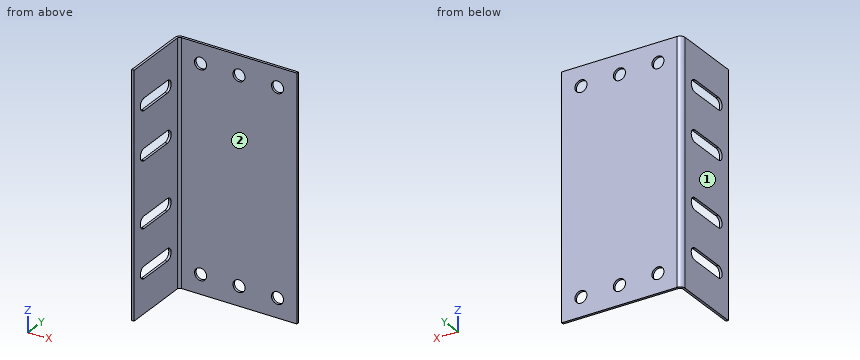
from build123d import *

# Parameters (mm, degrees)
BASE_FLANGE1_DEPTH = 100
CUT_EXTRUDE3_REACH = 117.758
SKETCH8_R          = 2.5
CUT_EXTRUDE4_REACH = 117.758
SKETCH11_R         = 2.5


# Sheet-metal steps are written as plain solids
with BuildPart() as part:
    # Sketch2 → Base-Flange1 (new body)
    with BuildSketch(Plane.XY):
        with BuildLine():
            Line((0, 0), (0, 28))
            ThreePointArc((0, 28), (0.585786438, 29.414213562), (2, 30))
            Line((2, 30), (50, 30))
            Line((50, 30), (50, 29))
            Line((50, 29), (2, 29))
            ThreePointArc((2, 29), (1.292893219, 28.707106781), (1, 28))
            Line((1, 28), (1, 0))
            Line((1, 0), (0, 0))
        make_face()
    extrude(amount=BASE_FLANGE1_DEPTH)

    # Sketch8 → Cut-Extrude3 (cut, up to next)
    with BuildSketch(Plane(origin=(0, 30, 0), x_dir=(1, 0, 0), z_dir=(0, 1, 0)), mode=Mode.PRIVATE) as cut_extrude3_sk1:
        with Locations(Location((42, -8, 0), (0, 0, 270))):
            Circle(SKETCH8_R)
    cut_extrude3_tool1 = extrude(cut_extrude3_sk1.sketch, amount=-CUT_EXTRUDE3_REACH, mode=Mode.PRIVATE) & part.part
    # Sketch8 → Cut-Extrude3 (cut, up to next)
    with BuildSketch(Plane(origin=(0, 30, 0), x_dir=(1, 0, 0), z_dir=(0, 1, 0)), mode=Mode.PRIVATE) as cut_extrude3_sk2:
        with Locations(Location((10, -8, 0), (0, 0, 270))):
            Circle(SKETCH8_R)
    cut_extrude3_tool2 = extrude(cut_extrude3_sk2.sketch, amount=-CUT_EXTRUDE3_REACH, mode=Mode.PRIVATE) & part.part
    # Sketch8 → Cut-Extrude3 (cut, up to next)
    with BuildSketch(Plane(origin=(0, 30, 0), x_dir=(1, 0, 0), z_dir=(0, 1, 0)), mode=Mode.PRIVATE) as cut_extrude3_sk3:
        with Locations(Location((42, -92, 0), (0, 0, 270))):
            Circle(SKETCH8_R)
    cut_extrude3_tool3 = extrude(cut_extrude3_sk3.sketch, amount=-CUT_EXTRUDE3_REACH, mode=Mode.PRIVATE) & part.part
    # Sketch8 → Cut-Extrude3 (cut, up to next)
    with BuildSketch(Plane(origin=(0, 30, 0), x_dir=(1, 0, 0), z_dir=(0, 1, 0)), mode=Mode.PRIVATE) as cut_extrude3_sk4:
        with Locations(Location((10, -92, 0), (0, 0, 270))):
            Circle(SKETCH8_R)
    cut_extrude3_tool4 = extrude(cut_extrude3_sk4.sketch, amount=-CUT_EXTRUDE3_REACH, mode=Mode.PRIVATE) & part.part
    # Sketch8 → Cut-Extrude3 (cut, up to next)
    with BuildSketch(Plane(origin=(0, 30, 0), x_dir=(1, 0, 0), z_dir=(0, 1, 0)), mode=Mode.PRIVATE) as cut_extrude3_sk5:
        with Locations(Location((26, -8, 0), (0, 0, 270))):
            Circle(SKETCH8_R)
    cut_extrude3_tool5 = extrude(cut_extrude3_sk5.sketch, amount=-CUT_EXTRUDE3_REACH, mode=Mode.PRIVATE) & part.part
    # Sketch8 → Cut-Extrude3 (cut, up to next)
    with BuildSketch(Plane(origin=(0, 30, 0), x_dir=(1, 0, 0), z_dir=(0, 1, 0)), mode=Mode.PRIVATE) as cut_extrude3_sk6:
        with Locations(Location((26, -92, 0), (0, 0, 270))):
            Circle(SKETCH8_R)
    cut_extrude3_tool6 = extrude(cut_extrude3_sk6.sketch, amount=-CUT_EXTRUDE3_REACH, mode=Mode.PRIVATE) & part.part
    add(cut_extrude3_tool1.solids().sort_by_distance((42, 30, 8))[0], mode=Mode.SUBTRACT)
    add(cut_extrude3_tool2.solids().sort_by_distance((10, 30, 8))[0], mode=Mode.SUBTRACT)
    add(cut_extrude3_tool3.solids().sort_by_distance((42, 30, 92))[0], mode=Mode.SUBTRACT)
    add(cut_extrude3_tool4.solids().sort_by_distance((10, 30, 92))[0], mode=Mode.SUBTRACT)
    add(cut_extrude3_tool5.solids().sort_by_distance((26, 30, 8))[0], mode=Mode.SUBTRACT)
    add(cut_extrude3_tool6.solids().sort_by_distance((26, 30, 92))[0], mode=Mode.SUBTRACT)

    # Sketch11 → Cut-Extrude4 (cut, up to next)
    with BuildSketch(Plane.ZY, mode=Mode.PRIVATE) as cut_extrude4_sk1:
        with BuildLine():
            ThreePointArc((19, 21.5), (16.5, 24), (14, 21.5))
            Line((14, 21.5), (14, 13.999999995))
            ThreePointArc((14, 13.999999995), (16.499999997, 16.5), (19, 14))
            Line((19, 14), (19, 21.5))
        make_face()
    cut_extrude4_tool1 = extrude(cut_extrude4_sk1.sketch, amount=-CUT_EXTRUDE4_REACH, mode=Mode.PRIVATE) & part.part
    # Sketch11 → Cut-Extrude4 (cut, up to next)
    with BuildSketch(Plane.ZY, mode=Mode.PRIVATE) as cut_extrude4_sk2:
        with BuildLine():
            ThreePointArc((19, 14), (16.500000003, 11.5), (14, 13.999999995))
            Line((14, 13.999999995), (14, 6.5))
            ThreePointArc((14, 6.5), (16.5, 4), (19, 6.5))
            Line((19, 6.5), (19, 14))
        make_face()
    cut_extrude4_tool2 = extrude(cut_extrude4_sk2.sketch, amount=-CUT_EXTRUDE4_REACH, mode=Mode.PRIVATE) & part.part
    # Sketch11 → Cut-Extrude4 (cut, up to next)
    with BuildSketch(Plane.ZY, mode=Mode.PRIVATE) as cut_extrude4_sk3:
        with Locations((16.5, 14)):
            Circle(SKETCH11_R)
    cut_extrude4_tool3 = extrude(cut_extrude4_sk3.sketch, amount=-CUT_EXTRUDE4_REACH, mode=Mode.PRIVATE) & part.part
    # Sketch11 → Cut-Extrude4 (cut, up to next)
    with BuildSketch(Plane.ZY, mode=Mode.PRIVATE) as cut_extrude4_sk4:
        with BuildLine():
            ThreePointArc((39, 14), (36.5, 11.5), (34, 14))
            Line((34, 14), (34, 6.5))
            ThreePointArc((34, 6.5), (36.5, 4), (39, 6.5))
            Line((39, 6.5), (39, 14))
        make_face()
    cut_extrude4_tool4 = extrude(cut_extrude4_sk4.sketch, amount=-CUT_EXTRUDE4_REACH, mode=Mode.PRIVATE) & part.part
    # Sketch11 → Cut-Extrude4 (cut, up to next)
    with BuildSketch(Plane.ZY, mode=Mode.PRIVATE) as cut_extrude4_sk5:
        with Locations((36.5, 14)):
            Circle(SKETCH11_R)
    cut_extrude4_tool5 = extrude(cut_extrude4_sk5.sketch, amount=-CUT_EXTRUDE4_REACH, mode=Mode.PRIVATE) & part.part
    # Sketch11 → Cut-Extrude4 (cut, up to next)
    with BuildSketch(Plane.ZY, mode=Mode.PRIVATE) as cut_extrude4_sk6:
        with BuildLine():
            ThreePointArc((39, 21.5), (36.5, 24), (34, 21.5))
            Line((34, 21.5), (34, 14))
            ThreePointArc((34, 14), (36.5, 16.5), (39, 14))
            Line((39, 14), (39, 21.5))
        make_face()
    cut_extrude4_tool6 = extrude(cut_extrude4_sk6.sketch, amount=-CUT_EXTRUDE4_REACH, mode=Mode.PRIVATE) & part.part
    # Sketch11 → Cut-Extrude4 (cut, up to next)
    with BuildSketch(Plane.ZY, mode=Mode.PRIVATE) as cut_extrude4_sk7:
        with BuildLine():
            Line((86, 14), (86, 21.5))
            ThreePointArc((86, 21.5), (83.5, 24), (81, 21.5))
            Line((81, 21.5), (81, 14))
            ThreePointArc((81, 14), (83.5, 16.5), (86, 14))
        make_face()
    cut_extrude4_tool7 = extrude(cut_extrude4_sk7.sketch, amount=-CUT_EXTRUDE4_REACH, mode=Mode.PRIVATE) & part.part
    # Sketch11 → Cut-Extrude4 (cut, up to next)
    with BuildSketch(Plane.ZY, mode=Mode.PRIVATE) as cut_extrude4_sk8:
        with BuildLine():
            Line((86, 6.5), (86, 14))
            ThreePointArc((86, 14), (83.5, 11.5), (81, 14))
            Line((81, 14), (81, 6.5))
            ThreePointArc((81, 6.5), (83.5, 4), (86, 6.5))
        make_face()
    cut_extrude4_tool8 = extrude(cut_extrude4_sk8.sketch, amount=-CUT_EXTRUDE4_REACH, mode=Mode.PRIVATE) & part.part
    # Sketch11 → Cut-Extrude4 (cut, up to next)
    with BuildSketch(Plane.ZY, mode=Mode.PRIVATE) as cut_extrude4_sk9:
        with Locations((83.5, 14)):
            Circle(SKETCH11_R)
    cut_extrude4_tool9 = extrude(cut_extrude4_sk9.sketch, amount=-CUT_EXTRUDE4_REACH, mode=Mode.PRIVATE) & part.part
    # Sketch11 → Cut-Extrude4 (cut, up to next)
    with BuildSketch(Plane.ZY, mode=Mode.PRIVATE) as cut_extrude4_sk10:
        with BuildLine():
            ThreePointArc((66, 21.5), (63.5, 24), (61, 21.5))
            Line((61, 21.5), (61, 14))
            ThreePointArc((61, 14), (63.5, 16.5), (66, 14))
            Line((66, 14), (66, 21.5))
        make_face()
    cut_extrude4_tool10 = extrude(cut_extrude4_sk10.sketch, amount=-CUT_EXTRUDE4_REACH, mode=Mode.PRIVATE) & part.part
    # Sketch11 → Cut-Extrude4 (cut, up to next)
    with BuildSketch(Plane.ZY, mode=Mode.PRIVATE) as cut_extrude4_sk11:
        with Locations((63.5, 14)):
            Circle(SKETCH11_R)
    cut_extrude4_tool11 = extrude(cut_extrude4_sk11.sketch, amount=-CUT_EXTRUDE4_REACH, mode=Mode.PRIVATE) & part.part
    # Sketch11 → Cut-Extrude4 (cut, up to next)
    with BuildSketch(Plane.ZY, mode=Mode.PRIVATE) as cut_extrude4_sk12:
        with BuildLine():
            ThreePointArc((66, 14), (63.5, 11.5), (61, 14))
            Line((61, 14), (61, 6.5))
            ThreePointArc((61, 6.5), (63.5, 4), (66, 6.5))
            Line((66, 6.5), (66, 14))
        make_face()
    cut_extrude4_tool12 = extrude(cut_extrude4_sk12.sketch, amount=-CUT_EXTRUDE4_REACH, mode=Mode.PRIVATE) & part.part
    add(cut_extrude4_tool1.solids().sort_by_distance((0, 19.713495, 16.5))[0], mode=Mode.SUBTRACT)
    add(cut_extrude4_tool2.solids().sort_by_distance((0, 8.286505, 16.5))[0], mode=Mode.SUBTRACT)
    add(cut_extrude4_tool3.solids().sort_by_distance((0, 14, 16.5))[0], mode=Mode.SUBTRACT)
    add(cut_extrude4_tool4.solids().sort_by_distance((0, 8.286505, 36.5))[0], mode=Mode.SUBTRACT)
    add(cut_extrude4_tool5.solids().sort_by_distance((0, 14, 36.5))[0], mode=Mode.SUBTRACT)
    add(cut_extrude4_tool6.solids().sort_by_distance((0, 19.713495, 36.5))[0], mode=Mode.SUBTRACT)
    add(cut_extrude4_tool7.solids().sort_by_distance((0, 19.713495, 83.5))[0], mode=Mode.SUBTRACT)
    add(cut_extrude4_tool8.solids().sort_by_distance((0, 8.286505, 83.5))[0], mode=Mode.SUBTRACT)
    add(cut_extrude4_tool9.solids().sort_by_distance((0, 14, 83.5))[0], mode=Mode.SUBTRACT)
    add(cut_extrude4_tool10.solids().sort_by_distance((0, 19.713495, 63.5))[0], mode=Mode.SUBTRACT)
    add(cut_extrude4_tool11.solids().sort_by_distance((0, 14, 63.5))[0], mode=Mode.SUBTRACT)
    add(cut_extrude4_tool12.solids().sort_by_distance((0, 8.286505, 63.5))[0], mode=Mode.SUBTRACT)


solid = part.part
Read the model definition and answer for the solid it produces. Units are mm, in the model's axes. Face numbers are marked on the shaded views. A direction names the side the tool comes from. Round coordinates to 2 decimals unless told otherwise and drop trailing zeros. Order: outer loops, then holes, each group sorted by start corner. A loop starts at its lowest first (then second) coordinate and runs counter-clockwise, first axis right, second up.
1) The part is cut by section A-A on z = 63.5. Write down the section's boundary in (x, y), plus the area to 3 significant figures.
2) The part is cut by section C-C on z = 8. Write down the section's boundary in (x, y).
3) The part is cut by section D-D on x = 42. Write down the section's boundary in (y, z).
4) Flat-ended cylindrical pins translate along their axes: pin 1 (2 mm diameter, centred on y = 7, z = 65.5, fed in from +X); pin 2 (4 mm diameter, centred on x = 26, z = 92, fed in from +Y); pin 3 (8 mm diameter, centred on x = 26, z = 8, fed in from -Y). Find the tip coordinate at first contact, or state that the pin passes through.
5) The part is cut by section B-B on y = 11.25. Write down the section's boundary in (x, z), plus the area to 3 significant figures.
6) For the marked faces 1 and 2, determine the directions among +Z, -Z, +X, -X, +Y, -Y from which every point of the face is accessible in a straight line to the end or side of a thin tool.
7) Straight lines are drawn through the part: L1, parallel to X at y = 29.65, z = 92; L2, parallel to X at y = 29.4, z = 92; L3, parallel to Y at x = 14, z = 65. For each, find the intervals that lie inside material, in ascending order.
Resolved:
1. outline: (0, 0) - (1, 0) - (1, 4) - (0, 4) - close; (0, 24) - (1, 24) - (1, 28) arc R1 cw to (2, 29) - (50, 29) - (50, 30) - (2, 30) arc R2 ccw to (0, 28) - close
1. area: 58.4 mm2
2. outline: (0, 0) - (1, 0) - (1, 28) arc R1 cw to (2, 29) - (7.5, 29) - (7.5, 30) - (2, 30) arc R2 ccw to (0, 28) - close; (12.5, 29) - (23.5, 29) - (23.5, 30) - (12.5, 30) - close; (28.5, 29) - (39.5, 29) - (39.5, 30) - (28.5, 30) - close; (44.5, 29) - (50, 29) - (50, 30) - (44.5, 30) - close
3. outline: (29, 0) - (30, 0) - (30, 5.5) - (29, 5.5) - close; (29, 10.5) - (30, 10.5) - (30, 89.5) - (29, 89.5) - close; (29, 94.5) - (30, 94.5) - (30, 100) - (29, 100) - close
4. pin 1: stops at x = 1
4. pin 2: passes through
4. pin 3: stops at y = 29
5. outline: (0, 0) - (1, 0) - (1, 14) - (0, 14) - close; (0, 19) - (1, 19) - (1, 34) - (0, 34) - close; (0, 39) - (1, 39) - (1, 61) - (0, 61) - close; (0, 66) - (1, 66) - (1, 81) - (0, 81) - close; (0, 86) - (1, 86) - (1, 100) - (0, 100) - close
5. area: 80.0 mm2
6. face 1: +Z, -Z, -X, +Y, -Y
6. face 2: +Z, -Z, +X, -Y
7. L1: x = 0.87 to 7.5, 12.5 to 23.5, 28.5 to 39.5, 44.5 to 50
7. L2: x = 0.57 to 7.5, 12.5 to 23.5, 28.5 to 39.5, 44.5 to 50
7. L3: y = 29 to 30
